Can you work these out from the model? Positions are in its coordinate system, mm. Face numbers are marked on the shaded views. Give positions to 0.01 mm unless a question says otherwise; leave off trailing zeros. Order: outer loops, then holes, each group sorted by start corner. A loop starts at its lowest first (then second) coordinate and runs counter-clockwise, first axis right, second up. Notation, with made-up numbers: (43.25, 27.25) - (49.25, 27.25) arc R17 ccw to (49.25, 42.25) - close; hole circle Ø5 at (33.5, 35). An arc over 180 degrees is marked (long way). Answer as a JSON object with one key per item and string values.
```python
from build123d import *

# Parameters (mm, degrees)
ESBO_O1_W                = 10
ESBO_O1_H                = 130
ESBO_O1_R                = 2.5
RESSALTO_EXTRUS_O1_DEPTH = 3
ESBO_O1_11_R             = 2.5
RESSALTO_EXTRUS_O7_DEPTH = 8


with BuildPart() as part:
    # Esboço1 → Ressalto-extrusão1 (new body)
    with BuildSketch(Plane.XY):
        Rectangle(ESBO_O1_W, ESBO_O1_H)
        with Locations((0, 55)):
            Circle(ESBO_O1_R, mode=Mode.SUBTRACT)
        with Locations((0, -60)):
            Circle(ESBO_O1_R, mode=Mode.SUBTRACT)
        with Locations((0, -25)):
            Circle(ESBO_O1_R, mode=Mode.SUBTRACT)
    extrude(amount=RESSALTO_EXTRUS_O1_DEPTH)

    # Esboço1<11> → Ressalto-extrusão7 (add)
    with BuildSketch(Plane.XY):
        with Locations((0, -25)):
            Circle(ESBO_O1_11_R)
        with Locations((0, -60)):
            Circle(ESBO_O1_11_R)
    extrude(amount=RESSALTO_EXTRUS_O7_DEPTH)


solid = part.part
```
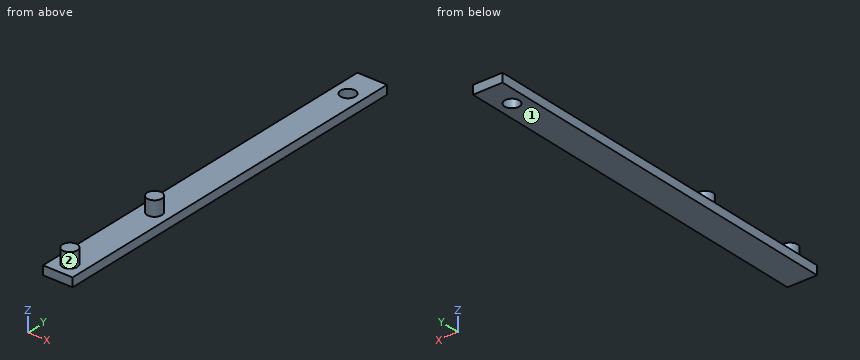
Q1. I need wall thicknesses on L1, parallel to Y at x = 0, z = 0.8; L2, parallel to Y at x = 0, z = 7.25; L3, parallel to Z at x = 0, y = -35.5. Which ranges of each line are inside material? Lowest first, please.
Recorded:
{"L1": "y = -65 to 52.5, 57.5 to 65", "L2": "y = -62.5 to -57.5, -27.5 to -22.5", "L3": "z = 0 to 3"}
Q2. If we section it at B-B, the plane z = 5.5: Please give me the cut outline in (x, y).
Recorded:
{"outline": "circle Ø5 at (0, -60); circle Ø5 at (0, -25)"}
Q3. We'd pull the mould along Y, two halves only. Please class the marked faces 1 and 2: released by +Y, released by -Y, zero draft, split by the parting line, or undercut.
Recorded:
{"face 1": "zero draft", "face 2": "undercut"}
Q4. I'm going to push flat-ended pins straight in: pin 1 Ø3 at (x, z) = (0.5, 6.5) entering from -Y; pin 2 Ø3 at (x, z) = (0.5, 6) entering from +Y; pin 3 Ø4 at (x, y) = (-2, 42.5) entering from +Z. Where does each tip first touch, or does it pass through?
Recorded:
{"pin 1": "stops at y = -62.5", "pin 2": "stops at y = -22.5", "pin 3": "stops at z = 3"}
Q5. If we section it at D-D, the plane y = -53: Please give me the cut outline in (x, z).
Recorded:
{"outline": "(-5, 0) - (5, 0) - (5, 3) - (-5, 3) - close"}
Q6. If we section it at C-C, the plane y = -25: Please give me the cut outline in (x, z), then the cut area to 3 significant figures.
Recorded:
{"outline": "(-5, 0) - (5, 0) - (5, 3) - (2.5, 3) - (2.5, 8) - (-2.5, 8) - (-2.5, 3) - (-5, 3) - close", "area": "55.0 mm^2"}
Q7. If we section it at A-A, the plane x = 0: Please give me the cut outline in (y, z), then the cut area to 3 significant figures.
Recorded:
{"outline": "(-65, 0) - (52.5, 0) - (52.5, 3) - (-22.5, 3) - (-22.5, 8) - (-27.5, 8) - (-27.5, 3) - (-57.5, 3) - (-57.5, 8) - (-62.5, 8) - (-62.5, 3) - (-65, 3) - close; (57.5, 0) - (65, 0) - (65, 3) - (57.5, 3) - close", "area": "425 mm^2"}
